from build123d import *

# Parameters (mm, degrees)
ESQUISSE1_R        = 4.5
BOSS_EXTRU_1_DEPTH = 8


with BuildPart() as part:
    # Esquisse1 → Boss.-Extru.1 (new body)
    # profile 1 of 2: a face of its own
    with BuildSketch(Plane(origin=(0, 0, 0), x_dir=(1, 0, 0), z_dir=(0, 1, 0))):
        Polygon((-190, 75), (-190, 0), (0, 0), (0, 90), (-90, 90), (-105, 75), align=None)
        with Locations(Location((-175, 20.5, 0), (0, 0, 270))):
            Circle(ESQUISSE1_R, mode=Mode.SUBTRACT)
        with Locations(Location((-140, 14, 0), (0, 0, 270))):
            Circle(ESQUISSE1_R, mode=Mode.SUBTRACT)
        with Locations(Location((-140, 34, 0), (0, 0, 270))):
            Circle(ESQUISSE1_R, mode=Mode.SUBTRACT)
        with Locations(Location((-175, 60.5, 0), (0, 0, 270))):
            Circle(ESQUISSE1_R, mode=Mode.SUBTRACT)
    # profile 2 of 2: a face of its own
    with BuildSketch(Plane(origin=(0, 0, 0), x_dir=(1, 0, 0), z_dir=(0, 1, 0))):
        Polygon((0, 90), (0, 0), (190, 0), (190, 75), (105, 75), (90, 90), align=None)
        with Locations(Location((140, 14, 0), (0, 0, 270))):
            Circle(ESQUISSE1_R, mode=Mode.SUBTRACT)
        with Locations(Location((175, 20.5, 0), (0, 0, 270))):
            Circle(ESQUISSE1_R, mode=Mode.SUBTRACT)
        with Locations(Location((140, 34, 0), (0, 0, 270))):
            Circle(ESQUISSE1_R, mode=Mode.SUBTRACT)
        with Locations(Location((175, 60.5, 0), (0, 0, 270))):
            Circle(ESQUISSE1_R, mode=Mode.SUBTRACT)
    extrude(amount=BOSS_EXTRU_1_DEPTH)


solid = part.part
For this review, take the finished solid that the model builds, in its own axes (mm). A direction names the side the tool comes from. Round coordinates to 2 decimals unless told otherwise and drop trailing zeros. Order: outer loops, then holes, each group sorted by start corner. A loop starts at its lowest first (then second) coordinate and runs counter-clockwise, first axis right, second up. Notation, with made-up numbers: (54.25, -2) -> (78.25, -2) arc R10 cw to (78.25, 4) -> close; hole circle Ø7 at (9.25, 56.5). An arc over 180 degrees is marked (long way). Write item = value, one per line. Start each with the question number.
1) Tool access review of faces 1 (the face through (171.01, 3.94, -58.42)), 2 (the face through (148, 4, -75)): name each direction out of +Z, -Z, +X, -X, +Y, -Y from which nothing blocks a thin tool from reaching the whole face with its end or side.
2) Take a section at D-D on z = -80.5. State the section outline as (x, y) points.
3) The part is to be moulded in two halves that separate along X. For faces 3 (the face through (-178.99, 3.94, -58.42)), 4 (the face through (190, 4, -37)), 5 (the face through (-147, 4, -75)), 6 (the face through (-190, 4, -38)), say which applies: +X half, -X half, draft (parallel to the pull), parting line (faces both ways), or undercut.
4) Take a section at A-A on z = -60.5. State the section outline as (x, y) points.
5) To check wall thickness, follow line 1 (X direction, y = 5.5, z = -60.5); line 2 (X direction, y = 7.75, z = -34); line 3 (Z direction, x = 141, y = 2.5). State the ranges of each line that lie inside material, in increasing order. Write a range as from..to.
6) Take a section at B-B on x = -140. State the section outline as (y, z) points, plus the area to 3 significant figures.
7) Insertion check: pin 1 (2.5 mm diameter, centred on x = 133.5, y = 5.5, fed in from -Z). The pin has a flat end and moves straight along its axis. Give the tip position at first contact, or say it passes through.
8) Take a section at C-C on y = 3. Count the separate pieces of the cut face and the enclosed holes in it, plus the area to 3 significant figures.
Verdict:
q1.face_1 = +Y, -Y
q1.face_2 = -Z, +X, +Y, -Y
q2.outline = (-99.5, 0) -> (99.5, 0) -> (99.5, 8) -> (-99.5, 8) -> close
q3.face_3 = undercut
q3.face_4 = +X half
q3.face_5 = draft
q3.face_6 = -X half
q4.outline = (-190, 0) -> (-179.5, 0) -> (-179.5, 8) -> (-190, 8) -> close; (-170.5, 0) -> (170.5, 0) -> (170.5, 8) -> (-170.5, 8) -> close; (179.5, 0) -> (190, 0) -> (190, 8) -> (179.5, 8) -> close
q5.line_1 = -190..-179.5, -170.5..170.5, 179.5..190
q5.line_2 = -190..-144.5, -135.5..135.5, 144.5..190
q5.line_3 = -75..-38.39, -29.61..-18.39, -9.61..0
q6.outline = (0, -75) -> (8, -75) -> (8, -38.5) -> (0, -38.5) -> close; (0, -29.5) -> (8, -29.5) -> (8, -18.5) -> (0, -18.5) -> close; (0, -9.5) -> (8, -9.5) -> (8, 0) -> (0, 0) -> close
q6.area = 456 mm2
q7.pin_1 = -75
q8.separate_pieces = 1
q8.enclosed_holes = 8
q8.area = 30,900 mm2
